The model under review builds one solid part; all positions refer to its coordinate system, in mm. Round coordinates to 2 decimals unless told otherwise and drop trailing zeros. Order: outer loops, then holes, each group sorted by start corner. A loop starts at its lowest first (then second) coordinate and runs counter-clockwise, first axis right, second up.
1) Consider section A-A (x = 15). Give the boundary of the cut face in (y, z).
2) Mouldability with a two-part tool opening along Z and no side actions: class faces 1 (the face through (0, 20, 20)), 2 (the face through (43.6, 27.5, 25.7)), 3 (the face through (35, 20, 0)) as pulls with the +Z half, pulls with the -Z half, needs draft (parallel to the pull), parting line crosses it, or undercut.
3) Consider section B-B (z = 4). Give the boundary of the cut face in (x, y), then the cut area to 3 significant figures.
4) Clearance check with flat-ended pins moving along their axes: P1, Ø8, axis at y = 27, z = 8, coming from the +X side; P2, Ø12, axis at x = 44.5, y = 36, coming from the +Z side. State where each tip first meets the part, or that it passes through.
5) To check wall thickness, follow L1, parallel to X at y = 23.5, z = 21.5; L2, parallel to Y at x = 30.5, z = 7.5; L3, parallel to Y at x = 25, z = 30. State the ranges of each line that lie inside material, in increasing order.
Autodesk Inventor part; units mm, degrees
ref_plane "工作平面1" through (70, 20, 20) normal (0.3333, 0.6667, 0.6667) x (-0.8944, 0.4472, 0)
ref_plane "YZ Plane" through (0, 0, 0) normal (1, 0, 0) x (0, 1, 0)
ref_plane "XZ Plane" through (0, 0, 0) normal (0, 1, 0) x (-1, 0, 0)
sketch "草圖5" plane through (0, 0, 0) normal (0, 0, 1) x (1, 0, 0)
  line L0 (0, 0) -> (70, 0)
  line L1 (70, 0) -> (70, 40)
  line L2 (70, 40) -> (0, 40)
  line L3 (0, 40) -> (0, 0)
  dimension "d20" = 70
  dimension "d21" = 40
extrude "擠出5" add sketch "草圖5" along normal blind 40
chamfer "倒角2" distance 20 distance2 40 1 edges at (70, 40, 20) measured on face at (70, 13.3333, 13.3333)
chamfer "倒角3" distance 20 distance2 20 1 edges at (15, 40, 40) measured on face at (33.3333, 13.3333, 40)
chamfer "倒角4" distance 40 distance2 20 1 edges at (70, 10, 40) measured on face at (23.3333, 13.3333, 40)
ref_plane "工作平面1" through (70, 20, 20) normal (0.3333, 0.6667, 0.6667) x (-0.8944, 0.4472, 0)
sketch "草圖9" plane through (70, 20, 20) normal (0.3333, 0.6667, 0.6667) x (-0.8944, 0.4472, 0)
  point P0 (53.6656, 17.8885)
sketch "草圖10" plane through (70, 20, 20) normal (0.3333, 0.6667, 0.6667) x (-0.8944, 0.4472, 0)
  line L0 (44.7214, -14.9071) -> (44.7214, 0)
  line L1 (44.7214, 0) -> (0, 0)
  line L2 (53.6656, 17.8885) -> (-8.9443, -2.9814)
  line L3 (0, 0) -> (35.7302, 26.9735)
  line L4 (44.7214, 0) -> (71.5542, 8.9443)
  line L5 (35.7302, 26.9735) -> (44.7214, 0)
extrude "擠出8" cut sketch "草圖10" along normal through all
Answer below:
1. outline: (0, 0) - (40, 0) - (40, 20) - (20, 40) - (0, 40) - close
2. face 1: needs draft
2. face 2: pulls with the +Z half
2. face 3: pulls with the -Z half
3. outline: (0, 0) - (70, 0) - (70, 20) - (30, 40) - (0, 40) - close
3. area: 2,400 mm2
4. P1: stops at x = 64
4. P2: stops at z = 23.46
5. L1: x = 0 to 60
5. L2: y = 0 to 39.75
5. L3: y = 0 to 30
